```python
from build123d import *

# Parameters (mm, degrees)
PAD_DEPTH    = 6.5
SKETCH001_R  = 2
POCKET_DEPTH = 5.701
FILLET_R     = 1


with BuildPart() as part:
    # Sketch → Pad (new body)
    with BuildSketch(Plane.XZ):
        Polygon((0, 0), (11.5, 0), (11.5, 5.7), (5, 5.7), (5, 4), (0, 4), align=None)
    extrude(amount=PAD_DEPTH)

    # Sketch001 → Pocket (cut, through all)
    with BuildSketch(Plane(origin=(0, 0, 5.7), x_dir=(-1, 0, 0), z_dir=(0, 0, 1))):
        with Locations((-8.25, 3.25)):
            Circle(SKETCH001_R)
    extrude(amount=-POCKET_DEPTH, mode=Mode.SUBTRACT)

    # Fillet
    fillet_edges = [part.edges().sort_by_distance(p)[0] for p in [
        (0, 0, 2),
        (0, -6.5, 2),
        (11.5, 0, 2.85),
        (11.5, -6.5, 2.85),
    ]]
    fillet(fillet_edges, radius=FILLET_R)


solid = part.part
```
Part model, mm, in its own coordinate system. Give positions to 0.01 mm unless a question says otherwise; leave off trailing zeros. Write each loop counter-clockwise with the first axis right and the second up, starting at its lowest first coordinate (ties: lowest second). Pieces come first, ordered by that corner, then holes. Notation, with made-up numbers: M 22,58.25 L 40,58.25 A17 ccw 40,80.25 Z; hole C 58.5,-13.5 d6. An arc over 180 degrees is marked long. Use CSV: the item, a comma, the result in double quotes.
Item 1: Slice it at D-D on y = -1.5. Write the cut outline in (x, z).
Taken from the geometry:
outline,"M 0,0 L 7.28,0 L 7.28,5.7 L 5,5.7 L 5,4 L 0,4 Z; M 9.22,0 L 11.5,0 L 11.5,5.7 L 9.22,5.7 Z"
Item 2: Slice it at B-B on y = -3.25. Write the cut outline in (x, z).
Taken from the geometry:
outline,"M 0,0 L 6.25,0 L 6.25,5.7 L 5,5.7 L 5,4 L 0,4 Z; M 10.25,0 L 11.5,0 L 11.5,5.7 L 10.25,5.7 Z"
Item 3: Slice it at A-A on x = 8.25. Write the cut outline in (y, z), plus the area to 4 significant figures.
Taken from the geometry:
outline,"M -6.5,0 L -5.25,0 L -5.25,5.7 L -6.5,5.7 Z; M -1.25,0 L 0,0 L 0,5.7 L -1.25,5.7 Z"
area,"14.25 mm²"
Item 4: Drill centre lines: probe 1 along Y at (x, z) = (8.25, 2.8); probe 2 along X at (y, z) = (-3.25, 3.7); probe 3 along Z at (x, y) = (0.75, -2.5). Where is each one in solid material? Low to high.
Taken from the geometry:
probe 1,"y = -6.5 to -5.25, -1.25 to 0"
probe 2,"x = 0 to 6.25, 10.25 to 11.5"
probe 3,"z = 0 to 4"
Item 5: Pull direction X, two halves, no side cores. Call faces 1 (the face through (3, -3, 4)), 2 (the face through (5, -3, 5)), 3 (the face through (11.5, -3, 3)), 4 (the face through (9.837, -2.033, 2.89)): +X half, -X half, draft (parallel to the pull), parting line (faces both ways), or undercut.
Taken from the geometry:
face 1,"draft"
face 2,"-X half"
face 3,"+X half"
face 4,"undercut"
Item 6: Slice it at C-C on z = 0.8. Write the cut outline in (x, y).
Taken from the geometry:
outline,"M 0,-5.5 A1 ccw 1,-6.5 L 10.5,-6.5 A1 ccw 11.5,-5.5 L 11.5,-1 A1 ccw 10.5,0 L 1,0 A1 ccw 0,-1 Z; hole C 8.25,-3.25 d4"
Item 7: Pin check, flat tips, straight feed: P1, Ø0.8, axis at y = -3, z = 5, coming from the -X side; P2, Ø3, axis at x = 8.25, y = -3.25, coming from the -Z side; P3, Ø2.5, axis at x = 2.5, y = -3.5, coming from the +Z side. Stop position of each tip, or through.
Taken from the geometry:
P1,"stops at x = 5"
P2,"passes through"
P3,"stops at z = 4"
